Autodesk Inventor part; units mm, degrees
ref_plane "YZ Plane" through (0, 0, 0) normal (1, 0, 0) x (0, 1, 0)
ref_plane "XZ Plane" through (0, 0, 0) normal (0, 1, 0) x (-1, 0, 0)
ref_plane "XY Plane" through (0, 0, 0) normal (0, 0, 1) x (1, 0, 0)
sketch "Sketch1" plane through (0, 0, 0) normal (0, 1, 0) x (-1, 0, 0)
  line L0 (0, 0) -> (20.32, 0)
  line L1 (20.32, 0) -> (20.32, -140)
  line L2 (20.32, -140) -> (0, -140)
  line L3 (0, -140) -> (0, 0)
  dimension "d0" = 140
  dimension "d1" = 20.32
extrude "Extrusion1" add sketch "Sketch1" along normal blind 10.16
sketch "Sketch2" plane through (-20.32, 0, 0) normal (0, 0, 1) x (1, 0, 0)
  line L0 (4.445, 7.493) -> (15.875, 7.493)
  line L1 (15.875, 7.493) -> (15.875, 2.667)
  line L2 (15.875, 2.667) -> (4.445, 2.667)
  line L3 (4.445, 2.667) -> (4.445, 7.493)
  line L4 (0, 10.16) -> (20.32, 10.16)
  line L5 (0, 0) -> (20.32, 0)
  line L6 (0, 0) -> (0, 10.16)
  line L7 (20.32, 0) -> (20.32, 10.16)
  line L8 (0, 10.16) -> (20.32, 10.16)
  line L9 (20.32, 10.16) -> (20.32, 0)
  line L10 (20.32, 0) -> (0, 0)
  line L11 (0, 0) -> (0, 10.16)
  dimension "d4" = 4.826
  dimension "d5" = 11.43
  dimension "d6" = 2.667
  dimension "d7" = 2.667
  dimension "d8" = 4.445
  dimension "d9" = 4.445
extrude "Extrusion2" cut sketch "Sketch2" against normal blind 10.16
sketch "Sketch3" plane through (0, 0, -140) normal (0, 0, -1) x (-1, 0, 0)
  line L0 (4.445, 7.493) -> (15.875, 7.493)
  line L1 (15.875, 2.667) -> (4.445, 2.667)
  line L2 (4.445, 7.493) -> (15.875, 7.493)
  line L3 (15.875, 7.493) -> (15.875, 2.667)
  line L4 (15.875, 2.667) -> (4.445, 2.667)
  line L5 (4.445, 2.667) -> (4.445, 7.493)
  line L6 (20.32, 0) -> (20.32, 10.16)
  line L7 (0, 10.16) -> (0, 0)
  line L8 (20.32, 10.16) -> (0, 10.16)
  line L9 (0, 10.16) -> (0, 0)
  line L10 (0, 0) -> (20.32, 0)
  line L11 (20.32, 0) -> (20.32, 10.16)
extrude "Extrusion3" cut sketch "Sketch3" against normal blind 10.16
equation "\"d6\" = d7"
equation "\"d8\" = d9"
properties part number "spool holder span" material "PLA"
Part model, mm, in its own coordinate system. A direction names the side the tool comes from. Round coordinates to 2 decimals unless told otherwise and drop trailing zeros. Write each loop counter-clockwise with the first axis right and the second up, starting at its lowest first coordinate (ties: lowest second). Pieces come first, ordered by that corner, then holes. Notation, with made-up numbers: M 50,-4 L 91,-4 A13 ccw 91,17 Z; hole C -1.75,65 d9. An arc over 180 degrees is marked long. Return JSON: item names as keys, results as strings. Group by question number.
(1) Saw through at C-C on x = -2.75. Write the cut outline in (y, z), then the cut area to 3 significant figures.
(2) Pin check, flat tips, straight feed: pin 1 Ø2.5 at (y, z) = (6, -135.5) entering from +X (3 decimals); pin 2 Ø3 at (x, z) = (-12, -136.5) entering from -Y; pin 3 Ø3 at (x, z) = (-10.5, -7.5) entering from +Y. Stop position of each tip, or through.
(3) Saw through at B-B on y = 6. Write the cut outline in (x, z) (3 decimals).
(4) Which spindle directions (+Z, -Z, +X, -X, +Y, -Y) get a long thin tool onto all of the face, cutting with end or side? Do faces 4 (the face through (-10, 2.667, -135)), 5 (the face through (-10, 7.493, -5)), 6 (the face through (-4.445, 5, -135)), 7 (the face through (-10, 2.667, -5)). Say none if no direction does.
(5) Drill centre line: probe 1 along Z at (x, y) = (-15.5, 2.25). Where is it in solid material? Low to high.
(6) Saw through at A-A on x = -13.5. Write the cut outline in (y, z).
(7) Two-plate mould, pull along X, no slides. Class faces 1 (the face through (-20.32, 5, -69)), 2 (the face through (-4.445, 5, -5)), 3 (the face through (-10, 5, -140)): +X half, -X half, draft (parallel to the pull), parting line (faces both ways), or undercut.
Returned:
{
 "1": {"outline": "M 0,-129.84 L 10.16,-129.84 L 10.16,-10.16 L 0,-10.16 Z", "area": "1,220 mm²"},
 "2": {"pin 1": "x = -4.445", "pin 2": "y = 2.67", "pin 3": "y = 7.49"},
 "3": {"outline": "M -20.32,-129.84 L -15.875,-129.84 L -15.875,-140 L -4.445,-140 L -4.445,-129.84 L 0,-129.84 L 0,-10.16 L -4.445,-10.16 L -4.445,0 L -15.875,0 L -15.875,-10.16 L -20.32,-10.16 Z"},
 "4": {"face 4": "-Z, +X, -X, -Y", "face 5": "+Z, +X, -X, +Y", "face 6": "-Z, +X, +Y, -Y", "face 7": "+Z, +X, -X, -Y"},
 "5": {"probe 1": "-129.84 to -10.16"},
 "6": {"outline": "M 0,-129.84 L 2.67,-129.84 L 2.67,-140 L 7.49,-140 L 7.49,-129.84 L 10.16,-129.84 L 10.16,-10.16 L 7.49,-10.16 L 7.49,0 L 2.67,0 L 2.67,-10.16 L 0,-10.16 Z"},
 "7": {"face 1": "-X half", "face 2": "+X half", "face 3": "draft"}
}
